Geometry check sheet. Reference: the model listing, model coordinates, mm. Give positions to 0.01 mm unless a question says otherwise; leave off trailing zeros. Order: outer loops, then holes, each group sorted by start corner. A loop starts at its lowest first (then second) coordinate and runs counter-clockwise, first axis right, second up.
```python
from build123d import *

# Parameters (mm, degrees)
BOSS_EXTRUDE1_DEPTH = 6.5
TAP1_D              = 6.647


with BuildPart() as part:
    # Sketch1 → Boss-Extrude1 (new body)
    with BuildSketch(Plane(origin=(0, 0, 0), x_dir=(0, 0, -1), z_dir=(1, 0, 0))):
        Polygon((6.5, -3.75277675), (6.5, 3.75277675), (0, 7.505553499), (-6.5, 3.75277675), (-6.5, -3.75277675), (0, -7.505553499), align=None)
    extrude(amount=BOSS_EXTRUDE1_DEPTH)

    # Sketch2 → Cut-Revolve1 (revolve, cut)
    with BuildSketch(Plane.XY):
        Polygon((6.5, 7.505553499), (6.5, 6.5), (5.919443416, 7.505553499), align=None)
        Polygon((0, 7.505553499), (0.580556584, 7.505553499), (0, 6.5), align=None)
    revolve(axis=Axis((-0.325, 0, 0), (1, 0, 0)), mode=Mode.SUBTRACT)

    # Tap1 (through all)
    with Locations(Plane(origin=(0, 0, 0), x_dir=(0, 0, -1), z_dir=(-1, 0, 0))):
        with Locations((0, 0)):
            Hole(TAP1_D / 2)


solid = part.part
```
Q1. Cross-section at A-A, the plane x = 5. Record the boundary of the cut face in (y, z).
Q2. Release check for a two-part mould opening along Z. For faces 1 (the face through (6.36, 3.36, -5.85)), 2 (the face through (3, 0, 6.5)), 3 (the face through (3.3, 1.27, 3.07)) record: pulls with the +Z half, pulls with the -Z half, needs draft (parallel to the pull), parting line crosses it, or undercut.
Q3. Gauge pin test, flat ends, axial feed: P1, Ø3, axis at x = 1.5, z = -5, coming from the +Y side; P2, Ø5.5, axis at y = 0, z = 0, coming from the +X side. Record the tip position at first contact, or that the pin passes through.
Q4. Thickness scan on L1, parallel to Z at x = 5.25, y = 3; L2, parallel to Z at x = 5.25, y = -2; L3, parallel to Z at x = 1, y = -5.5. Record the ranges inside material, lowest first.
Answers follow:
1. outline: (-7.51, 0) - (-3.75, -6.5) - (3.75, -6.5) - (7.51, 0) - (3.75, 6.5) - (-3.75, 6.5) - close; hole circle Ø6.65 at (0, 0)
2. face 1: pulls with the -Z half
2. face 2: pulls with the +Z half
2. face 3: undercut
3. P1: stops at y = 5.48
3. P2: passes through
4. L1: z = -6.5 to -1.43, 1.43 to 6.5
4. L2: z = -6.5 to -2.65, 2.65 to 6.5
4. L3: z = -3.47 to 3.47
